Design review of the part built by this model. Coordinates are the model's own, in mm. Face numbers are marked on the shaded views. A direction names the side the tool comes from. Round coordinates to 2 decimals unless told otherwise and drop trailing zeros. Loops run counter-clockwise (first coordinate to the right, second up) from the corner with the lowest first, then second, coordinate; pieces in that order, holes last. Notation, with made-up numbers: (67, 7.25) - (119, 7.25) arc R19 cw to (119, 23.25) - close; hole circle Ø9 at (-3, 17). An arc over 180 degrees is marked (long way). One line per question, with ' | ' between items. Start each with the question number.
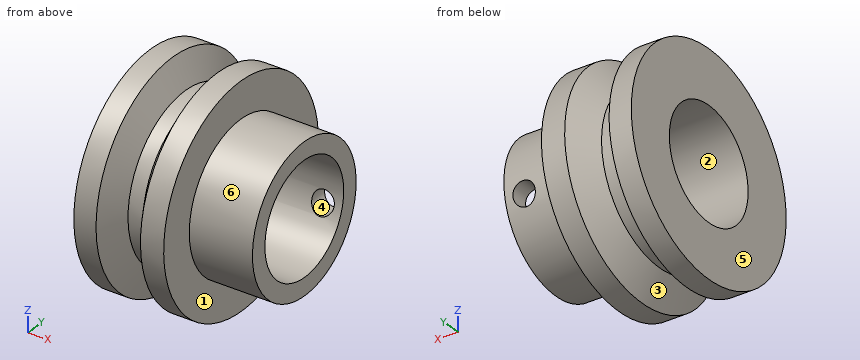
from build123d import *

# Parameters (mm, degrees)
SKETCH1_W          = 201.666666667
SKETCH1_H          = 73.666666667
SKETCH9_R          = 75
CUT_EXTRUDE1_DEPTH = 294.471179732
SKETCH14_R         = 15
CUT_EXTRUDE4_DEPTH = 268.773118171


with BuildPart() as part:
    # Sketch1 → Revolve4 (revolve)
    with BuildSketch(Plane.XY, mode=Mode.PRIVATE) as revolve4_sk:
        with Locations((-36.632641292, 36.833333334)):
            Rectangle(SKETCH1_W, SKETCH1_H)
        Polygon((-112.465974625, 147.333333333), (-142.465974625, 147.333333333), (-142.465974625, 0), (-137.465974625, 0), (-137.465974625, 73.666666667), (64.200692042, 73.666666667), (64.200692042, 98.666666667), (-21.132641292, 98.666666667), (-21.132641292, 147.333333333), (-52.465974625, 147.333333333), (-75.799307958, 110), (-95.799307958, 110), align=None)
    revolve(revolve4_sk.sketch.rotate(Axis((-184.465974625, 0, 0), (1, 0, 0)), 90), axis=Axis((-184.465974625, 0, 0), (1, 0, 0)))

    # Sketch9 → Cut-Extrude1 (cut, through all)
    with BuildSketch(Plane.ZY.offset(142.465974625)):
        Circle(SKETCH9_R)
    extrude(amount=-CUT_EXTRUDE1_DEPTH, mode=Mode.SUBTRACT)

    # Sketch14 → Cut-Extrude4 (cut, through all)
    with BuildSketch(Plane(origin=(0, 25, 0), x_dir=(1, 0, 0), z_dir=(0, 1, 0))):
        with Locations(Location((38.628593536, 21.914529815, 0), (0, 0, 90))):
            Circle(SKETCH14_R)
    extrude(amount=CUT_EXTRUDE4_DEPTH, mode=Mode.SUBTRACT)


solid = part.part
1. Take a section at C-C, the plane x = 43. Give the boundary of the cut face in (y, z).
2. Machinability: for the marked faces 1, 2 and 3, which of the approach directions +Z, -Z, +X, -X, +Y, -Y give a long, thin tool a straight path to every point of the face, cutting with its end or side? Answer none if there is none.
3. Take a section at D-D, the plane z = -29.5. Count the separate pieces of the cut face and the enclosed holes in it, then the cut area to 3 significant figures.
4. Take a section at A-A, the plane y = 0. Give the boundary of the cut face in (x, z).
5. To check wall thickness, follow line 1 along Y through (x, z) = (-123.5, -3.5); line 2 along Y through (x, z) = (-46.5, 0); line 3 along Z through (x, y) = (-72, -66). State the ranges of each line that lie inside material, in increasing order.
6. Clearance check with flat-ended pins moving along their axes: P1, Ø12, axis at x = 21.5, z = 87.5, coming from the -Y side; P2, Ø18, axis at x = 38.63, z = -21.91, coming from the +Y side; P3, Ø8, axis at x = -26.5, z = -103, coming from the +Y side; P4, Ø10, axis at y = 100, z = 18, coming from the +X side. State where each tip first meets the part, or that it passes through.
7. The part is to be moulded in two halves that separate along Z. For the marked faces 4, 5 and 6, say which applies: pulls with the +Z half, pulls with the -Z half, needs draft (parallel to the pull), parting line crosses it, or undercut.
Answer list:
1) outline: (65.65, -36.26) arc R75 cw (long way) to (74.62, -7.57) - (98.38, -7.57) arc R98.67 ccw (long way) to (91.76, -36.26) - close
2) face 1: +X | face 2: +X, -X | face 3: none
3) separate pieces: 3 | enclosed holes: 0 | area: 18,900 mm²
4) outline: (-142.47, -147.33) - (-112.47, -147.33) - (-95.8, -110) - (-75.8, -110) - (-52.47, -147.33) - (-21.13, -147.33) - (-21.13, -98.67) - (64.2, -98.67) - (64.2, -75) - (-142.47, -75) - close; (-142.47, 75) - (64.2, 75) - (64.2, 98.67) - (-21.13, 98.67) - (-21.13, 147.33) - (-52.47, 147.33) - (-75.8, 110) - (-95.8, 110) - (-112.47, 147.33) - (-142.47, 147.33) - close
5) line 1: y = -147.29 to -74.92, 74.92 to 147.29 | line 2: y = -147.33 to -75, 75 to 147.33 | line 3: z = -95.49 to -35.62, 35.62 to 95.49
6) P1: stops at y = -55.61 | P2: stops at y = -68.33 | P3: stops at y = 109.12 | P4: stops at x = 64.2
7) face 4: undercut | face 5: needs draft | face 6: parting line crosses it
